Check sheet for the modelled part. Datum: model origin and axes. Units: mm. A direction names the side the tool comes from. Round coordinates to 2 decimals unless told otherwise and drop trailing zeros. Loops run counter-clockwise (first coordinate to the right, second up) from the corner with the lowest first, then second, coordinate; pieces in that order, holes last. Notation, with made-up numbers: M 84.25,4.25 L 92.25,4.25 A22 cw 92.25,21.25 Z; hole C 6,-22.75 d8. An arc over 180 degrees is marked long. Write item = value, one per line. Start each with the question number.
(1) Go/stop test with flat-tipped pins: P1, Ø10, axis at y = -29, z = 5, coming from the -X side; P2, Ø6, axis at y = -6.5, z = 9, coming from the +X side; P3, Ø8, axis at x = -4, z = 18.5, coming from the +Y side. Record where each tip stops, or that it passes through.
(2) Scan lines: L1, parallel to Y at x = 0, z = 2.2; L2, parallel to X at y = -65, z = 4.25; L3, parallel to Z at x = -82.5, y = 44.5. Record each from-to range of solid material in increasing order. Write a range as from..to.
(3) Set-up check for faces 1 (the face through (95, 0, 23)), 2 (the face through (0.59, -90.54, 13.87)): record each of +Z, -Z, +X, -X, +Y, -Y from which the full face is reachable in a straight line by a thin tool's end or side.
(4) Mould release check, pull along Y, two halves, no side actions. Record for faces 3 (the face through (0.59, 99.46, 13.87)), 4 (the face through (-90.504, 0.198, 13.874)), 5 (the face through (-95, 0, 23)): pulls with the +Y half, pulls with the -Y half, needs draft (parallel to the pull), parting line crosses it, or undercut.
(5) Cross-section at D-D on y = -56.5. Record the boundary of the cut face in (x, z).
(6) Cross-section at A-A on y = 0. Record the boundary of the cut face in (x, z), plus the area to 3 significant figures.
(7) Cross-section at C-C on z = 8.75. Record the boundary of the cut face in (x, y).
Autodesk Fusion 360 part; units mm, degrees
sketch "Sketch1" plane through (0, 0, 0) normal (0, 0, 1) x (1, 0, 0)
  circle A0 centre (0, 0) radius 100
  circle A1 centre (0, 0) radius 90
  dimension "d1" = 200
  dimension "d2" = 180
extrude "Extrude1" add sketch "Sketch1" along normal blind 5
sketch "Sketch2" plane through (0, 0, 5) normal (0, 0, 1) x (-1, 0, 0)
  circle A0 centre (0, 0) radius 90
  circle A1 centre (0, 0) radius 100
  line L0 (0, 0) -> (-95, 0) construction
  line L1 (-95, 0) -> (95, 0) construction
  line L2 (95, 0) -> (95, -95) construction
  line L3 (95, -95) -> (-95, -95) construction
  line L4 (-95, -95) -> (-95, 0) construction
  line L5 (-95, 0) -> (95, 0) construction
  line L6 (95, 0) -> (95, 95) construction
  line L7 (95, 95) -> (-95, 95) construction
  line L8 (-95, 95) -> (-95, 0) construction
  circle A2 centre (95, 0) radius 4.5
  circle A3 centre (0, -95) radius 4.5
  circle A4 centre (-95, 0) radius 4.5
  circle A5 centre (0, 95) radius 4.5
  dimension "d5" = 95
  dimension "d6" = 190
  dimension "d7" = 95
  dimension "d8" = 190
  dimension "d9" = 95
  dimension "d10" = 9
  dimension "d11" = 9
  dimension "d12" = 9
  dimension "d13" = 9
extrude "Extrude2" add sketch "Sketch2" along normal blind 18 contours A2 | A3 | A4 | A5
Result:
q1.P1 = -97.08
q1.P2 = 97.83
q1.P3 = 99.5
q2.L1 = -100..-90, 90..100
q2.L2 = -75.99..-62.25, 62.25..75.99
q2.L3 = 0..5
q3.face_1 = +Z, +X, -X, +Y, -Y
q3.face_2 = +Z
q4.face_3 = undercut
q4.face_4 = parting line crosses it
q4.face_5 = needs draft
q5.outline = M -82.51,0 L -70.06,0 L -70.06,5 L -82.51,5 Z; M 70.06,0 L 82.51,0 L 82.51,5 L 70.06,5 Z
q6.outline = M -100,0 L -90,0 L -90,5 L -90.5,5 L -90.5,23 L -99.5,23 L -99.5,5 L -100,5 Z; M 90,0 L 100,0 L 100,5 L 99.5,5 L 99.5,23 L 90.5,23 L 90.5,5 L 90,5 Z
q6.area = 424 mm^2
q7.outline = C -95,0 d9; C 0,-95 d9; C 0,95 d9; C 95,0 d9
